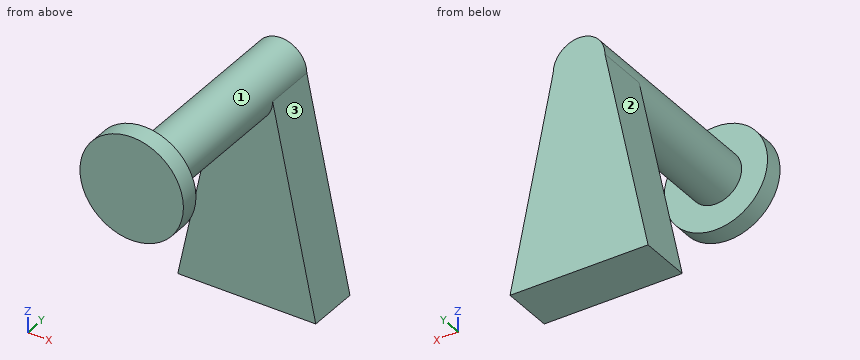
from build123d import *

# Parameters (mm, degrees)
F1_DEPTH = 609.6
F2_DEPTH = 152.4
F3_R     = 152.4
F4_DEPTH = 55.88


with BuildPart() as f1:
    # F0 (on Front) → F1 (new body)
    with BuildSketch(Plane.XZ):
        with BuildLine():
            ThreePointArc((-76.2, 0), (0, -76.2), (76.2, 0))
            ThreePointArc((76.2, 0), (0, 76.2), (-76.2, 0))
        make_face()
    extrude(amount=F1_DEPTH)

    # F0 (on Front) → F2 (join)
    with BuildSketch(Plane.XZ):
        with BuildLine():
            Line((203.2, -609.6), (76.2, 0))
            ThreePointArc((76.2, 0), (0, -76.2), (-76.2, 0))
            Line((-76.2, 0), (-203.2, -609.6))
            Line((-203.2, -609.6), (203.2, -609.6))
        make_face()
    extrude(amount=F2_DEPTH)

    # F3 (on face) → F4 (join)
    with BuildSketch(Plane.XZ.offset(609.6)):
        Circle(F3_R)
    extrude(amount=F4_DEPTH)


solid = f1.part
Work out the finished part from the listing and answer in its coordinate system (mm). Face numbers are marked on the shaded views. A direction names the side the tool comes from. Give positions to 0.01 mm unless a question says otherwise; leave off trailing zeros. Write each loop counter-clockwise with the first axis right and the second up, starting at its lowest first coordinate (ties: lowest second). Pieces come first, ordered by that corner, then holes.
Q1. The part is cut by section D-D on z = -301.5. Give the vertices of the cut face in (x, y).
Answer:
outline: (-139.01, -152.4) - (139.01, -152.4) - (139.01, 0) - (-139.01, 0) - close
Q2. Straight lines are drawn through the part: L1, parallel to Y at x = -2.5, z = -81; L2, parallel to Y at x = -127.5, z = -4.5; L3, parallel to Y at x = -50, z = -269.5. For each, find the intervals that lie inside material, in ascending order.
Answer:
L1: y = -665.48 to -609.6, -152.4 to 0
L2: y = -665.48 to -609.6
L3: y = -152.4 to 0
Q3. The part is cut by section A-A on x = 0. Give the vertices of the cut face in (y, z).
Answer:
outline: (-665.48, -152.4) - (-609.6, -152.4) - (-609.6, -76.2) - (-152.4, -76.2) - (-152.4, -609.6) - (0, -609.6) - (0, 76.2) - (-609.6, 76.2) - (-609.6, 152.4) - (-665.48, 152.4) - close
Q4. The part is cut by section B-B on x = 136. Give the vertices of the cut face in (y, z).
Answer:
outline: (-665.48, -68.77) - (-609.6, -68.77) - (-609.6, 68.77) - (-665.48, 68.77) - close; (-152.4, -609.6) - (0, -609.6) - (0, -287.04) - (-152.4, -287.04) - close
Q5. The part is cut by section C-C on y = -132. Give the vertices of the cut face in (x, z).
Answer:
outline: (-203.2, -609.6) - (203.2, -609.6) - (76.2, 0) arc R76.2 ccw to (-76.2, 0) - close
Q6. Given pin 1 (1 mm diameter, centred on y = -117, z = -296.5, fed in from +X) (3 decimals); pin 2 (6 mm diameter, centred on x = -17, y = -347.5, fed in from -Z); pin 3 (2 mm diameter, centred on x = 46.5, y = -425, fed in from -Z), each flat-ended and moving along its own axis, determine where each tip first touches the part or whether it passes through.
Answer:
pin 1: stops at x = 138.075
pin 2: stops at z = -74.9
pin 3: stops at z = -61.12
Q7. A tool of negligible diameter and unlimited length cuts with its end or side. For the marked faces 1, 2 and 3, from which of +Z, -Z, +X, -X, +Y, -Y can it reach the whole face along a straight path? Write none if from no direction.
Answer:
face 1: none
face 2: +Z, -X, +Y
face 3: +Z, +X, +Y
